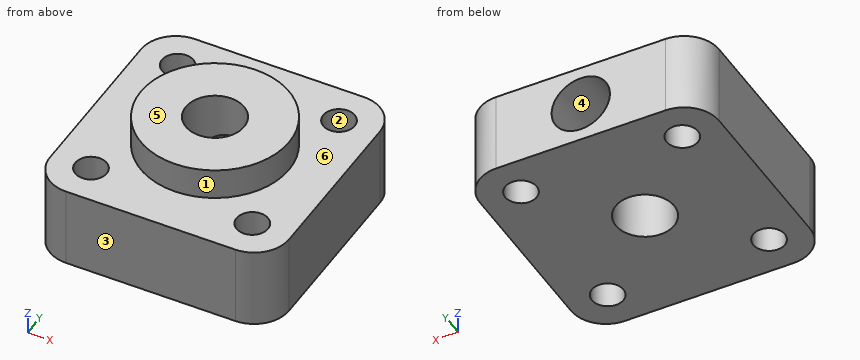
```python
from build123d import *

# Parameters (mm, degrees)
CROQUIS1_W              = 20.5
CROQUIS1_H              = 20.5
SALIENTE_EXTRUIR1_DEPTH = 7
REDONDEO1_R             = 3
CROQUIS2_R              = 6.35
SALIENTE_EXTRUIR2_DEPTH = 2.7
CROQUIS3_R              = 2.5
CORTAR_EXTRUIR1_DEPTH   = 10.7
CROQUIS4_R              = 1.35
CORTAR_EXTRUIR2_DEPTH   = 8
CORTAR_EXTRUIR3_REACH   = 22.5
CROQUIS5_R              = 2.5


with BuildPart() as part:
    # Croquis1 → Saliente-Extruir1 (new body)
    with BuildSketch(Plane.XY):
        Rectangle(CROQUIS1_W, CROQUIS1_H)
    extrude(amount=SALIENTE_EXTRUIR1_DEPTH)

    # Redondeo1
    redondeo1_edges = [part.edges().sort_by_distance(p)[0] for p in [
        (10.25, -10.25, 3.5),
        (-10.25, -10.25, 3.5),
        (-10.25, 10.25, 3.5),
        (10.25, 10.25, 3.5),
    ]]
    fillet(redondeo1_edges, radius=REDONDEO1_R)

    # Croquis2 → Saliente-Extruir2 (add)
    with BuildSketch(Plane.XY.offset(7)):
        Circle(CROQUIS2_R)
    extrude(amount=SALIENTE_EXTRUIR2_DEPTH)

    # Croquis3 → Cortar-Extruir1 (cut, through all)
    with BuildSketch(Plane.XY.offset(9.7)):
        Circle(CROQUIS3_R)
    extrude(amount=-CORTAR_EXTRUIR1_DEPTH, mode=Mode.SUBTRACT)

    # Croquis4 → Cortar-Extruir2 (cut, through all)
    with BuildSketch(Plane.XY.offset(7)):
        with Locations((-6.91550432, 6.91550432)):
            Circle(CROQUIS4_R)
        with Locations((6.91550432, 6.91550432)):
            Circle(CROQUIS4_R)
        with Locations((6.91550432, -6.91550432)):
            Circle(CROQUIS4_R)
        with Locations((-6.91550432, -6.91550432)):
            Circle(CROQUIS4_R)
    extrude(amount=-CORTAR_EXTRUIR2_DEPTH, mode=Mode.SUBTRACT)

    # Croquis5 → Cortar-Extruir3 (cut, up to next)
    with BuildSketch(Plane(origin=(0, 10.25, 0), x_dir=(1, 0, 0), z_dir=(0, 1, 0)), mode=Mode.PRIVATE) as cortar_extruir3_sk1:
        with Locations((0, -3.5)):
            Circle(CROQUIS5_R)
    cortar_extruir3_tool1 = extrude(cortar_extruir3_sk1.sketch, amount=-CORTAR_EXTRUIR3_REACH, mode=Mode.PRIVATE) & part.part
    add(cortar_extruir3_tool1.solids().sort_by_distance((0, 10.25, 3.5))[0], mode=Mode.SUBTRACT)


solid = part.part
```
For this review, take the finished solid that the model builds, in its own axes (mm). Face numbers are marked on the shaded views. A direction names the side the tool comes from. Round coordinates to 2 decimals unless told otherwise and drop trailing zeros. Loops run counter-clockwise (first coordinate to the right, second up) from the corner with the lowest first, then second, coordinate; pieces in that order, holes last.
(1) Mouldability with a two-part tool opening along Y and no side actions: class the marked faces 1, 2 and 3 as released by +Y, released by -Y, zero draft, split by the parting line, or undercut.
Returned:
face 1: split by the parting line
face 2: undercut
face 3: released by -Y
(2) We need section A-A (z = 3.5). Give the boundary of the cut face in (x, y).
Returned:
outline: (-10.25, -7.25) arc R3 ccw to (-7.25, -10.25) - (7.25, -10.25) arc R3 ccw to (10.25, -7.25) - (10.25, 7.25) arc R3 ccw to (7.25, 10.25) - (2.5, 10.25) - (2.5, 0) arc R2.5 cw to (-2.5, 0) - (-2.5, 10.25) - (-7.25, 10.25) arc R3 ccw to (-10.25, 7.25) - close; hole circle Ø2.7 at (-6.92, -6.92); hole circle Ø2.7 at (-6.92, 6.92); hole circle Ø2.7 at (6.92, -6.92); hole circle Ø2.7 at (6.92, 6.92)
(3) Tool access review of the marked faces 4, 5 and 6: name each direction out of +Z, -Z, +X, -X, +Y, -Y from which nothing blocks a thin tool from reaching the whole face with its end or side.
Returned:
face 4: +Y
face 5: +Z, +X, -X, +Y, -Y
face 6: +Z
(4) We need section C-C (y = -0.25). Give the boundary of the cut face in (x, z).
Returned:
outline: (-10.25, 0) - (-2.49, 0) - (-2.49, 9.7) - (-6.35, 9.7) - (-6.35, 7) - (-10.25, 7) - close; (2.49, 0) - (10.25, 0) - (10.25, 7) - (6.35, 7) - (6.35, 9.7) - (2.49, 9.7) - close
(5) Wall thickness on line 1 along Y through (x, z) = (7, 5); line 2 along X through (y, z) = (0, 3.25); line 3 along Y through (x, z) = (0, 9.25): over which ranges is each line inside the solid? List them lowest first.
Returned:
line 1: y = -10.25 to -8.26, -5.57 to 5.57, 8.26 to 10.25
line 2: x = -10.25 to -2.5, 2.5 to 10.25
line 3: y = -6.35 to -2.5, 2.5 to 6.35
(6) We need section B-B (x = 0.5). Give the boundary of the cut face in (y, z).
Returned:
outline: (-10.25, 0) - (-2.45, 0) - (-2.45, 9.7) - (-6.33, 9.7) - (-6.33, 7) - (-10.25, 7) - close; (2.45, 0) - (10.25, 0) - (10.25, 1.05) - (2.45, 1.05) - close; (2.45, 5.95) - (10.25, 5.95) - (10.25, 7) - (6.33, 7) - (6.33, 9.7) - (2.45, 9.7) - close
(7) Clearance check with flat-ended pins moving along their axes: P1, Ø3.5, axis at x = -6.92, y = 6.92, coming from the +Z side; P2, Ø1.6, axis at x = -6.92, y = -6.92, coming from the -Z side. State where each tip first meets the part, or that it passes through.
Returned:
P1: stops at z = 7
P2: passes through
(8) We need section D-D (z = 6.75). Give the boundary of the cut face in (x, y), plus the area to 3 significant figures.
Returned:
outline: (-10.25, -7.25) arc R3 ccw to (-7.25, -10.25) - (7.25, -10.25) arc R3 ccw to (10.25, -7.25) - (10.25, 7.25) arc R3 ccw to (7.25, 10.25) - (-7.25, 10.25) arc R3 ccw to (-10.25, 7.25) - close; hole circle Ø2.7 at (-6.92, -6.92); hole circle Ø2.7 at (-6.92, 6.92); hole circle Ø5 at (0, 0); hole circle Ø2.7 at (6.92, -6.92); hole circle Ø2.7 at (6.92, 6.92)
area: 370 mm2
